from build123d import *

# Parameters (mm, degrees)
F1_DEPTH = 25.4
F2_R     = 0.6


with BuildPart() as f1:
    # F0 (on Front) → F1 (new body)
    with BuildSketch(Plane.XZ):
        Polygon((9.3241402825, 8.2967067137), (0, 31.6984727979), (-10.0554463643, 8.2967067137), (-26.7336517572, 8.2967067137), (-10.0554463643, -5.155775696), (-17.8360161943, -23.2632836642), (0, -8.402004838), (16.2311457098, -23.2632836642), (9.3241402825, -5.155775696), (25.7989484817, 8.2967067137), align=None)
    extrude(amount=F1_DEPTH)

    # F2
    f2_edges = [f1.edges().sort_by_distance(p)[0] for p in [
        (4.66207, -25.4, 19.99759),
        (-5.027723, -25.4, 19.99759),
        (-18.394549, -25.4, 8.296707),
        (-18.394549, -25.4, 1.570466),
        (-13.945731, -25.4, -14.20953),
        (-8.918008, -25.4, -15.832644),
        (8.115573, -25.4, -15.832644),
        (12.777643, -25.4, -14.20953),
        (17.561544, -25.4, 1.570466),
        (17.561544, -25.4, 8.296707),
        (25.798948, -12.7, 8.296707),
        (9.32414, -12.7, 8.296707),
        (17.561544, 0, 8.296707),
        (0, -12.7, 31.698473),
        (4.66207, 0, 19.99759),
        (-10.055446, -12.7, 8.296707),
        (-5.027723, 0, 19.99759),
        (-10.055446, -12.7, -5.155776),
        (-17.836016, -12.7, -23.263284),
        (-13.945731, 0, -14.20953),
        (-26.733652, -12.7, 8.296707),
        (-18.394549, 0, 1.570466),
        (0, -12.7, -8.402005),
        (16.231146, -12.7, -23.263284),
        (8.115573, 0, -15.832644),
        (-8.918008, 0, -15.832644),
        (9.32414, -12.7, -5.155776),
        (17.561544, 0, 1.570466),
        (12.777643, 0, -14.20953),
        (-18.394549, 0, 8.296707),
    ]]
    fillet(f2_edges, radius=F2_R)


solid = f1.part
For this review, take the finished solid that the model builds, in its own axes (mm). A direction names the side the tool comes from. Give positions to 0.01 mm unless a question says otherwise; leave off trailing zeros. Write each loop counter-clockwise with the first axis right and the second up, starting at its lowest first coordinate (ties: lowest second). Pieces come first, ordered by that corner, then holes. Notation, with made-up numbers: (-37, -26.5) -> (20, -26.5) arc R26 ccw to (20, 8.5) -> close; hole circle Ø6 at (58.25, 6.25). An arc over 180 degrees is marked (long way). Use CSV: the item, a comma, the result in double quotes.
Q1. To check wall thickness, follow probe 1 along X at (y, z) = (-9.5, -19); probe 2 along X at (y, z) = (-1.25, 6.5); probe 3 along Z at (x, y) = (-20, -8.5). State the ranges of each line that lie inside material, in increasing order. Write a range as [from, to].
Conclusion:
probe 1,"[-16, -12.72], [11.57, 14.6]"
probe 2,"[-24.51, 23.6]"
probe 3,"[2.87, 8.3]"
Q2. Mouldability with a two-part tool opening along Z and no side actions: class faces 1 (the face through (-8.266, -12.531, -15.289)), 2 (the face through (17.07, -0.18, 1.39)), 3 (the face through (-5.17, -12.53, 19.67)) as pulls with the +Z half, pulls with the -Z half, needs draft (parallel to the pull), parting line crosses it, or undercut.
Conclusion:
face 1,"pulls with the -Z half"
face 2,"undercut"
face 3,"pulls with the +Z half"
Q3. Tool access review of faces 4 (the face through (7.277, -12.531, -15.064)), 5 (the face through (-13.43, -25.22, -13.44)), 6 (the face through (-17.7, -0.18, 1.23)), 7 (the face through (12.2, -25.22, -13.18)), 8 (the face through (17, -13, 8.297)): name each direction out of +Z, -Z, +X, -X, +Y, -Y from which nothing blocks a thin tool from reaching the whole face with its end or side.
Conclusion:
face 4,"-Z, +Y, -Y"
face 5,"-X, -Y"
face 6,"-X, +Y"
face 7,"+X, -Y"
face 8,"+Z, +X, +Y, -Y"
Q4. For P1, Ø8, axis at x = 19.5, y = -22.5, coming from the -Z side; P2, Ø12, axis at y = -15, z = -13, coming from the -X side; P3, Ø2, axis at y = -15, z = -1, coming from the -X side, all flat-tipped, find the tip position at first contact; note any pin that passes through.
Conclusion:
P1,"z = -0.11"
P2,"x = -16"
P3,"x = -16.45"
Q5. Take a section at A-A, the plane y = -3.25. Write out the cut boundary in (x, z), then the cut area to 3 significant figures.
Conclusion:
outline,"(-25.41, 7.23) -> (-10.41, -4.87) arc R0.6 cw to (-10.24, -5.57) -> (-16.85, -20.96) arc R0.6 ccw to (-15.91, -21.66) -> (-0.4, -8.74) arc R0.6 cw to (0.39, -8.76) -> (14.36, -21.55) arc R0.6 ccw to (15.33, -20.9) -> (9.48, -5.56) arc R0.6 cw to (9.66, -4.88) -> (24.49, 7.23) arc R0.6 ccw to (24.12, 8.3) -> (9.73, 8.3) arc R0.6 cw to (9.17, 8.67) -> (0.54, 30.35) arc R0.6 ccw to (-0.57, 30.37) -> (-9.9, 8.66) arc R0.6 cw to (-10.45, 8.3) -> (-25.03, 8.3) arc R0.6 ccw to start"
area,"938 mm2"
